Could you check a few things on this model? Use its own coordinates, in mm. Coordinates: 2 decimals unless noted, no trailing zeros. Order: outer loops, then holes, each group sorted by start corner. A loop starts at its lowest first (then second) coordinate and runs counter-clockwise, first axis right, second up. Notation, with made-up numbers: (80.25, 72.25) -> (118.25, 72.25) arc R22 ccw to (118.25, 81.25) -> close; hole circle Ø5 at (41.5, -9). An arc over 180 degrees is marked (long way). Put each result on its own line as item: value. Start each with the question number.
Q1. If we section it at B-B (x = -90.5): Please give me the cut outline in (y, z) (3 decimals), and give its area (3 significant figures).
Q2. Please list where these lines run through material, in increasing order: line 1 along X through (y, z) = (617.5, -1.5); line 2 along X through (y, z) = (90, 8.5); line 3 along Z through (x, y) = (-8, 83).
Q3. If we section it at A-A (y = 652.5): Please give me the cut outline in (x, z) (3 decimals).
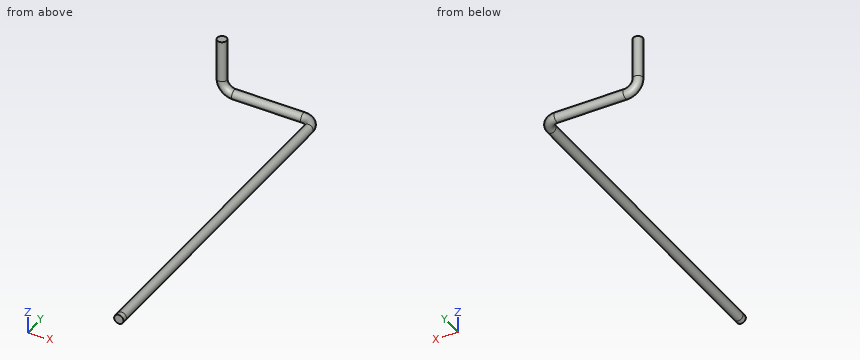
from build123d import *

# Parameters (mm, degrees)
CROQUIS1_R              = 9.525
SALIENTE_EXTRUIR1_DEPTH = 10
CROQUIS2_R              = 9.525


with BuildPart() as part:
    # Croquis1 → Saliente-Extruir1 (new body)
    with BuildSketch(Plane(origin=(0, 0, 0), x_dir=(1, 0, 0), z_dir=(0, 1, 0))):
        with Locations(Location((0, 0, 0), (0, 0, 270))):
            Circle(CROQUIS1_R)
    extrude(amount=SALIENTE_EXTRUIR1_DEPTH)

    # Barrer1: sweep along a curve in space
    with BuildLine() as barrer1_path:
        Line((0, 10, 0), (0, 665, 0))
        ThreePointArc((0, 665, 0), (-7.32233047, 682.67766953, 0), (-25, 690, 0))
        Line((-25, 690, 0), (-165, 690, 0))
        ThreePointArc((-165, 690, 0), (-182.67766953, 690, 7.32233047), (-190, 690, 25))
        Line((-190, 690, 25), (-190, 690, 110))
    # Croquis2 → Barrer1 (sweep)
    with BuildSketch(Plane(origin=(0, 10, 0), x_dir=(1, 0, 0), z_dir=(0, 1, 0))):
        Circle(CROQUIS2_R)
    sweep(path=barrer1_path.line)


solid = part.part
The answers:
1. outline: circle Ø19.05 at (690, 0)
1. area: 285 mm^2
2. line 1: -9.41 to 9.41
2. line 2: -4.3 to 4.3
2. line 3: -5.17 to 5.17
3. outline: circle Ø19.05 at (0, 0)
